Part model, mm, in its own coordinate system. A direction names the side the tool comes from. Give positions to 0.01 mm unless a question says otherwise; leave off trailing zeros. Write each loop counter-clockwise with the first axis right and the second up, starting at its lowest first coordinate (ties: lowest second). Pieces come first, ordered by that corner, then holes. Notation, with made-up numbers: M 71.5,61.5 L 125.5,61.5 A28 cw 125.5,80.5 Z; hole C -33.5,-35 d4. An arc over 180 degrees is marked long. Use a Markdown table: item, result. Add a question column.
from build123d import *

# Parameters (mm, degrees)
F0_W     = 10
F0_H     = 15
F1_DEPTH = 1.15
F2_W     = 10
F2_H     = 1.45
F2_R     = 0.575
F3_DEPTH = 1.85
F5_W     = 1.0999371812
F5_H     = 4.9819686796
F5_H_2   = 7.9447921516
F6_DEPTH = 16.3
F7_R     = 1
F8_DEPTH = 3


with BuildPart() as f1:
    # F0 (on Top) → F1 (new body)
    with BuildSketch(Plane.XY):
        with Locations((4.657e-07, -0.4447921516)):
            Rectangle(F0_W, F0_H)
    extrude(amount=F1_DEPTH)

    # F2 (on face) → F3 (join)
    with BuildSketch(Plane(origin=(0, 0, 0), x_dir=(1, 0, 0), z_dir=(0, 0, -1))):
        with Locations((4.657e-07, 0.4447921516)):
            Rectangle(F2_W, F2_H)
        with Locations((4.657e-07, -4.5802078484)):
            Circle(F2_R)
        with Locations((4.657e-07, 5.4697921516)):
            Circle(F2_R)
    extrude(amount=F3_DEPTH)

    # F5 (on face) → F6 (join)
    with BuildSketch(Plane.XY.offset(1.15)):
        with Locations((-3.14094e-05, -10.4357764914)):
            Rectangle(F5_W, F5_H)
        with Locations((-3.14094e-05, -3.9723960758)):
            Rectangle(F5_W, F5_H_2)
    extrude(amount=F6_DEPTH)

    # F7 (on face) → F8 (cut)
    with BuildSketch(Plane(origin=(-0.55, 0, 0), x_dir=(0, -1, 0), z_dir=(-1, 0, 0))):
        with BuildLine():
            Line((0, 17.45), (0, 1.15))
            Line((0, 1.15), (9.5370645307, 16.5871438408))
            ThreePointArc((9.5370645307, 16.5871438408), (10.109500032, 17.170324419), (10.8773304556, 17.45))
            Line((10.8773304556, 17.45), (0, 17.45))
        make_face()
        with BuildLine():
            Line((12.9267608312, 17.45), (11.3445362076, 17.45))
            ThreePointArc((11.3445362076, 17.45), (12.375279512, 16.9653370525), (12.9267608312, 15.9687437117))
            Line((12.9267608312, 15.9687437117), (12.9267608312, 17.45))
        make_face()
        with Locations((11.0667608312, 15.6007357099)):
            Circle(F7_R)
        with Locations((11.0667608312, 12.2007357099)):
            Circle(F7_R)
        with Locations((11.0667608312, 8.8007357099)):
            Circle(F7_R)
        with Locations((11.0667608312, 5.4007357099)):
            Circle(F7_R)
        with BuildLine():
            Line((7.9447921516, 2.1431122441), (7.9447921516, 1.15))
            Line((7.9447921516, 1.15), (12.9267608312, 1.15))
            Line((12.9267608312, 1.15), (12.9267608312, 4.15))
            Line((12.9267608312, 4.15), (12.9267608312, 5.1628855511))
            ThreePointArc((12.9267608312, 5.1628855511), (12.6698856531, 4.3234567709), (11.9872399284, 3.7715325472))
            Line((11.9872399284, 3.7715325472), (7.9447921516, 2.1431122441))
        make_face()
    extrude(amount=-F8_DEPTH, mode=Mode.SUBTRACT)


solid = f1.part
1. Drill centre lines: probe 1 along X at (y, z) = (-9.25, 16); probe 2 along Z at (x, y) = (2, 1); probe 3 along Y at (x, z) = (2.75, 0.75). Where is each one in solid material? Low to high. Write a range as [from, to].
2. Cut at C-C (x = 3.25). Write the cut outline in (y, z).
3. Tool access for faces 1 (the flat face through (-0.55, -8, 7)), 2 (the flat face through (0.55, -8, 7)), 3 (the flat face through (0, -7.945, 1)): list every direction of +Z, -Z, +X, -X, +Y, -Y with a clear straight run to the whole face (end or side of a thin tool).
4. Cut at D-D (z = 3). Write the cut outline in (x, y), then the cut area to 3 significant figures.
5. Cut at B-B (x = 0). Write the cut outline in (y, z).
6. Flat gauge pins, fed straight in: pin 1 (0.9 mm diameter, centred on x = 1.5, z = -0.5, fed in from +Y); pin 2 (2.5 mm diameter, centred on y = -11.07, z = 8.8, fed in from -X); pin 3 (5.5 mm diameter, centred on x = -1, y = -5.5, fed in from -Z); pin 4 (5 mm diameter, centred on y = -7, z = 8.5, fed in from +X). Where does each tip first touch, or does it go through?
7. Mould opens along Z. For faces 4 (the flat face through (0, 0.28, -1)), 5 (the cylindrical face through (-0.008, -10.068, 5.445)), 6 (the flat face through (0, 5, -1.85)) say: released by +Z, released by -Z, zero draft, split by the parting line, or undercut.
8. Cut at A-A (y = -4.5). Write the cut outline in (x, z), then the cut area to 3 significant figures.
A:
| question | item | result |
|---|---|---|
| 1 | probe 1 | x = [-0.55, 0.55] |
| 1 | probe 2 | z = [0, 1.15] |
| 1 | probe 3 | y = [-7.94, 7.06] |
| 2 | outline | M -7.94,0 L -1.17,0 L -1.17,-1.85 L 0.28,-1.85 L 0.28,0 L 7.06,0 L 7.06,1.15 L -7.94,1.15 Z |
| 3 | face 1 | +Z, -X, +Y, -Y |
| 3 | face 2 | +Z, +X, +Y, -Y |
| 3 | face 3 | -Z, +X, -X, -Y |
| 4 | outline | M -0.55,-10.07 L 0.55,-10.07 L 0.55,-1.14 L -0.55,-1.14 Z |
| 4 | area | 9.82 mm² |
| 5 | outline | M -12.93,5.16 A1.5 ccw -11.99,3.77 L -7.94,2.14 L -7.94,0 L -6.04,0 L -6.04,-1.85 L -4.89,-1.85 L -4.89,0 L -1.17,0 L -1.17,-1.85 L 0.28,-1.85 L 0.28,0 L 4.01,0 L 4.01,-1.85 L 5.16,-1.85 L 5.16,0 L 7.06,0 L 7.06,1.15 L 0,1.15 L -9.54,16.59 A1.85 ccw -10.88,17.45 L -11.34,17.45 A1.85 ccw -12.93,15.97 Z; hole C -11.07,5.4 d2; hole C -11.07,8.8 d2; hole C -11.07,12.2 d2; hole C -11.07,15.6 d2 |
| 6 | pin 1 | stops at y = 0.28 |
| 6 | pin 2 | stops at x = -0.55 |
| 6 | pin 3 | stops at z = -1.85 |
| 6 | pin 4 | stops at x = 0.55 |
| 7 | face 4 | zero draft |
| 7 | face 5 | undercut |
| 7 | face 6 | released by -Z |
| 8 | outline | M -5,0 L 5,0 L 5,1.15 L 0.55,1.15 L 0.55,8.43 L -0.55,8.43 L -0.55,1.15 L -5,1.15 Z |
| 8 | area | 19.5 mm² |
